Verification items for the finished model (mm, model axes). A direction names the side the tool comes from. Give positions to 0.01 mm unless a question says otherwise; leave off trailing zeros. Write each loop counter-clockwise with the first axis right and the second up, starting at its lowest first coordinate (ties: lowest second). Pieces come first, ordered by that corner, then holes. Notation, with made-up numbers: (-8.75, 45.5) - (37.25, 45.5) arc R13 ccw to (37.25, 65.5) - close; hole circle Ø11 at (54.5, 77). An arc over 180 degrees is marked (long way). Put each result on its own line as item: value.
from build123d import *

# Parameters (mm, degrees)
BOSS_EXTRUDE1_DEPTH = 71.26


with BuildPart() as part:
    # Loft13: read off the stored shape, not the designer's step
    # Loft13: loft between two sections, ruled curve by curve
    loft13_from = [
        Edge.make_bspline([(-79.603627765, 0, 56.755489551), (-76.115966153, 0, 64.213426555), (-72.628304542, 0, 71.67136356), (-65.652981318, 0, 86.587237568), (-62.165319707, 0, 94.045174572), (-58.677658095, 0, 101.503111577)], [0, 0, 0, 0, 0.5, 0.5, 1, 1, 1, 1], 3),
        Edge.make_bspline([(-58.677658095, 0, 101.503111577), (-48.906538694, 0, 103.830924441), (-39.135419292, 0, 106.158737306), (-19.59318049, 0, 110.814363034), (-9.822061088, 0, 113.142175899), (-0.050941687, 0, 115.469988763)], [0, 0, 0, 0, 0.5, 0.5, 1, 1, 1, 1], 3),
        Edge.make_bspline([(-74.603627765, 0, 56.755489551), (-75.436961098, 0, 56.755489551), (-76.270294432, 0, 56.755489551), (-77.936961098, 0, 56.755489551), (-78.770294432, 0, 56.755489551), (-79.603627765, 0, 56.755489551)], [0, 0, 0, 0, 0.5, 0.5, 1, 1, 1, 1], 3),
        Edge.make_bspline([(-0.050941687, 0, 115.469988763), (8.91697935, 0, 112.796539052), (17.884900386, 0, 110.12308934), (35.820742459, 0, 104.776189918), (44.788663496, 0, 102.102740206), (53.756584532, 0, 99.429290495)], [0, 0, 0, 0, 0.5, 0.5, 1, 1, 1, 1], 3),
        Edge.make_bspline([(53.756584532, 0, 99.429290495), (56.963215816, 0, 92.316990338), (60.1698471, 0, 85.20469018), (66.583109668, 0, 70.980089866), (69.789740951, 0, 63.867789708), (72.996372235, 0, 56.755489551)], [0, 0, 0, 0, 0.5, 0.5, 1, 1, 1, 1], 3),
        Edge.make_bspline([(72.996372235, 0, 56.755489551), (72.163038902, 0, 56.755489551), (71.329705568, 0, 56.755489551), (69.663038902, 0, 56.755489551), (68.829705568, 0, 56.755489551), (67.996372235, 0, 56.755489551)], [0, 0, 0, 0, 0.5, 0.5, 1, 1, 1, 1], 3),
        Edge.make_bspline([(67.996372235, 0, 56.755489551), (65.019950017, 0, 63.178013733), (62.043527798, 0, 69.600537914), (56.090683362, 0, 82.445586278), (53.114261143, 0, 88.86811046), (50.137838925, 0, 95.290634641)], [0, 0, 0, 0, 0.5, 0.5, 1, 1, 1, 1], 3),
        Edge.make_bspline([(50.137838925, 0, 95.290634641), (41.74895364, 0, 97.791466534), (33.360068355, 0, 100.292298427), (16.582297786, 0, 105.293962214), (8.193412501, 0, 107.794794107), (-0.195472784, 0, 110.295626)], [0, 0, 0, 0, 0.5, 0.5, 1, 1, 1, 1], 3),
        Edge.make_bspline([(-0.195472784, 0, 110.295626), (-9.358047044, 0, 108.112789279), (-18.520621304, 0, 105.929952558), (-36.845769825, 0, 101.564279116), (-46.008344086, 0, 99.381442395), (-55.170918346, 0, 97.198605674)], [0, 0, 0, 0, 0.5, 0.5, 1, 1, 1, 1], 3),
        Edge.make_bspline([(-55.170918346, 0, 97.198605674), (-58.409703249, 0, 90.45808632), (-61.648488152, 0, 83.717566966), (-68.126057959, 0, 70.236528259), (-71.364842862, 0, 63.496008905), (-74.603627765, 0, 56.755489551)], [0, 0, 0, 0, 0.5, 0.5, 1, 1, 1, 1], 3),
    ]
    loft13_to = [
        Edge.make_bspline([(-79.755478337, 22.698681281, 30), (-77.736400655, 24.717758964, 30), (-75.717322973, 26.736836646, 30), (-71.679167608, 30.774992011, 30), (-69.660089926, 32.794069693, 30), (-67.641012243, 34.813147375, 30)], [0, 0, 0, 0, 0.5, 0.5, 1, 1, 1, 1], 3),
        Edge.make_bspline([(-67.641012243, 34.813147375, 30), (-55.973275602, 34.813147375, 30), (-44.305538961, 34.813147375, 30), (-20.97006568, 34.813147375, 30), (-9.302329039, 34.813147375, 30), (2.365407602, 34.813147375, 30)], [0, 0, 0, 0, 0.5, 0.5, 1, 1, 1, 1], 3),
        Edge.make_bspline([(-74.755478337, 20.62761347, 30), (-75.588811671, 20.972791438, 30), (-76.422145004, 21.317969407, 30), (-78.088811671, 22.008325344, 30), (-78.922145004, 22.353503313, 30), (-79.755478337, 22.698681281, 30)], [0, 0, 0, 0, 0.5, 0.5, 1, 1, 1, 1], 3),
        Edge.make_bspline([(2.365407602, 34.813147375, 30), (12.09284893, 34.813147375, 30), (21.820290258, 34.813147375, 30), (41.275172913, 34.813147375, 30), (51.002614241, 34.813147375, 30), (60.730055569, 34.813147375, 30)], [0, 0, 0, 0, 0.5, 0.5, 1, 1, 1, 1], 3),
        Edge.make_bspline([(60.730055569, 34.813147375, 30), (62.749133251, 32.794069693, 30), (64.768210933, 30.774992011, 30), (68.806366298, 26.736836646, 30), (70.82544398, 24.717758964, 30), (72.844521663, 22.698681281, 30)], [0, 0, 0, 0, 0.5, 0.5, 1, 1, 1, 1], 3),
        Edge.make_bspline([(72.844521663, 22.698681281, 30), (72.011188329, 22.353503313, 30), (71.177854996, 22.008325344, 30), (69.511188329, 21.317969407, 30), (68.677854996, 20.972791438, 30), (67.844521663, 20.62761347, 30)], [0, 0, 0, 0, 0.5, 0.5, 1, 1, 1, 1], 3),
        Edge.make_bspline([(67.844521663, 20.62761347, 30), (66.313599345, 22.158535787, 30), (64.782677027, 23.689458105, 30), (61.720832392, 26.75130274, 30), (60.189910074, 28.282225058, 30), (58.658987757, 29.813147375, 30)], [0, 0, 0, 0, 0.5, 0.5, 1, 1, 1, 1], 3),
        Edge.make_bspline([(58.658987757, 29.813147375, 30), (47.117545897, 29.813147375, 30), (35.576104037, 29.813147375, 30), (12.493220317, 29.813147375, 30), (0.951778457, 29.813147375, 30), (-10.589663403, 29.813147375, 30)], [0, 0, 0, 0, 0.5, 0.5, 1, 1, 1, 1], 3),
        Edge.make_bspline([(-10.589663403, 29.813147375, 30), (-19.753043574, 29.813147375, 30), (-28.916423746, 29.813147375, 30), (-47.243184088, 29.813147375, 30), (-56.40656426, 29.813147375, 30), (-65.569944431, 29.813147375, 30)], [0, 0, 0, 0, 0.5, 0.5, 1, 1, 1, 1], 3),
        Edge.make_bspline([(-65.569944431, 29.813147375, 30), (-67.100866749, 28.282225058, 30), (-68.631789067, 26.75130274, 30), (-71.693633702, 23.689458105, 30), (-73.22455602, 22.158535787, 30), (-74.755478337, 20.62761347, 30)], [0, 0, 0, 0, 0.5, 0.5, 1, 1, 1, 1], 3),
    ]
    loft13 = Solid(Shell([*[Face.make_surface_from_curves(loft13_from[k], loft13_to[k]) for k in range(10)], Face(Wire(loft13_from)), Face(Wire(loft13_to))]))
    add(loft13)

    # Sketch9 → Boss-Extrude1 (add)
    with BuildSketch(Plane.XY.offset(30)):
        Polygon((-79.770999887, 22.67425966), (-74.770999887, 20.603191848), (-65.585465981, 29.788725754), (58.643466207, 29.788725754), (67.829000113, 20.603191848), (72.829000113, 22.67425966), (60.714534019, 34.788725754), (-67.656533793, 34.788725754), align=None)
    extrude(amount=-BOSS_EXTRUDE1_DEPTH)


solid = part.part
Q1. Set-up check for faces 4 (the face through (63.17, 25.26, -5.13)), 5 (the face through (-77.306, 21.653, -5.131)), 6 (the face through (70.294, 21.624, -5.131)): record each of +Z, -Z, +X, -X, +Y, -Y from which the full face is reachable in a straight line by a thin tool's end or side.
Answers follow:
face 4: -Z, -Y
face 5: -Z, -X, -Y
face 6: -Z, +X, -Y
Q2. Release check for a two-part mould opening along X. For faces 1 (the face through (66.857, 28.647, -5.131)), 2 (the face through (-5, 31, -41.26)), 3 (the face through (-70.243, 25.132, -5.131)) record: released by +X, released by -X, zero draft, split by the parting line, or undercut.
Answers follow:
face 1: released by +X
face 2: zero draft
face 3: undercut
Q3. Go/stop test with flat-tipped pins: pin 1 Ø6 at (y, z) = (27, 18) entering from +X; pin 2 Ø8 at (x, y) = (6, 23.5) entering from +Z; pin 3 Ø8 at (x, z) = (-20, -8.5) entering from -Y; pin 4 Ø9.5 at (x, y) = (-39.5, 27) entering from -Z. Record where each tip stops, or that it passes through.
Answers follow:
pin 1: stops at x = 71.5
pin 2: stops at z = 67.02
pin 3: stops at y = 29.79
pin 4: stops at z = -41.26
Q4. Section check A-A, the plane z = -0.5. Record the cut outline in (x, y), plus the area to 3 significant figures.
Answers follow:
outline: (-79.77, 22.67) - (-74.77, 20.6) - (-65.59, 29.79) - (58.64, 29.79) - (67.83, 20.6) - (72.83, 22.67) - (60.71, 34.79) - (-67.66, 34.79) - close
area: 782 mm2
Q5. Scan lines: line 1 along X through (y, z) = (28, -4); line 2 along X through (y, z) = (17.5, 45); line 3 along Y through (x, z) = (6, 14.5). Record each from-to range of solid material in increasing order.
Answers follow:
line 1: x = -74.45 to -67.37, 60.43 to 67.5
line 2: x = -74.3 to -68.2, 61.47 to 67.56
line 3: y = 29.79 to 34.79
